Input: dimensioned drawing with shaded views. Units: mm. Origin: part minimum x, y, z. Give positions to 0.01 mm unless a question says otherwise; leave off trailing zeros. Order: outer loops, then holes, each group sorted by start corner. A loop starts at its lowest first (then second) coordinate and runs counter-clockwise, first axis right, second up. Notation, with made-up numbers: M 52.25,80.5 L 69.25,80.5 A19 cw 69.25,95.5 Z; hole C 23,46 d4. An arc over 180 degrees is marked long. Answer in a Markdown table with one row per item. Add a question column.
(1) Section query A-A, the plane x = 22. Return loops of the section in (y, z).
(2) Material intervals for line 1 along Z through (x, y) = (22, 13.1); line 2 along Y through (x, z) = (6.75, 2); line 3 along X through (y, z) = (11.5, 6.25), sorted ascending.
(3) Pin query (flat end, axial travel): P1, Ø1.5, axis at y = 13, z = 4, coming from the -X side; P2, Ø2.5, axis at x = 19.5, z = 4, coming from the -Y side; P3, Ø2, axis at y = 4, z = 9, coming from the -X side; P4, Ø3, axis at y = 2.5, z = 7, coming from the -X side. Return the tip coordinate at first contact, or that it passes through.
(4) Section query D-D, the plane y = 11.75. Return loops of the section in (x, z), plus the area to 3 significant figures.
(5) Section query B-B, the plane z = 5. Return loops of the section in (x, y), plus the area to 3 significant figures.
(6) Section query C-C, the plane z = 3. Return loops of the section in (x, y).
(7) Mould query, pull axis X, two halves, no side actions, for the marked faces 1, 2, 3 and 4. Classes: pulls with the +X half, pulls with the -X half, needs draft (parallel to the pull), parting line crosses it, or undercut.
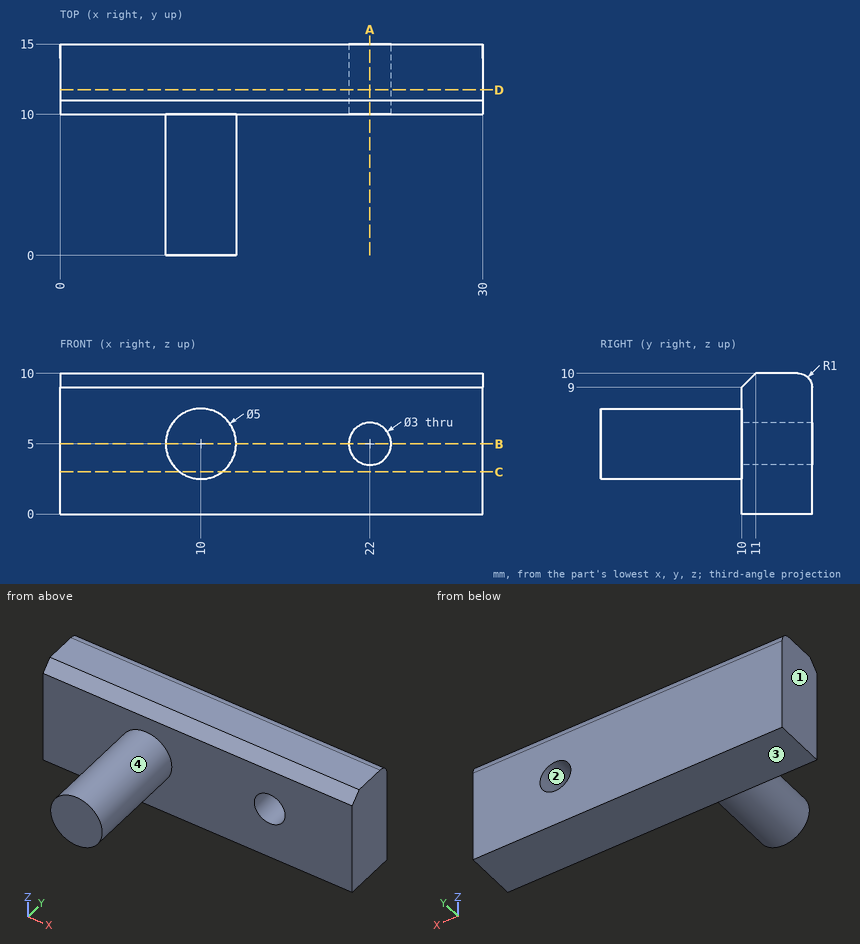
Values follow:
| question | item | result |
|---|---|---|
| 1 | outline | M 10,0 L 15,0 L 15,3.5 L 10,3.5 Z; M 10,6.5 L 15,6.5 L 15,9 A1 ccw 14,10 L 11,10 L 10,9 Z |
| 2 | line 1 | z = 0 to 3.5, 6.5 to 10 |
| 2 | line 2 | y = 10 to 15 |
| 2 | line 3 | x = 0 to 21.17, 22.83 to 30 |
| 3 | P1 | stops at x = 0 |
| 3 | P2 | stops at y = 10 |
| 3 | P3 | passes through |
| 3 | P4 | stops at x = 7.55 |
| 4 | outline | M 0,0 L 30,0 L 30,10 L 0,10 Z; hole C 22,5 d3 |
| 4 | area | 293 mm² |
| 5 | outline | M 0,10 L 7.5,10 L 7.5,0 L 12.5,0 L 12.5,10 L 20.5,10 L 20.5,15 L 0,15 Z; M 23.5,10 L 30,10 L 30,15 L 23.5,15 Z |
| 5 | area | 185 mm² |
| 6 | outline | M 0,10 L 8.5,10 L 8.5,0 L 11.5,0 L 11.5,10 L 30,10 L 30,15 L 0,15 Z |
| 7 | face 1 | pulls with the -X half |
| 7 | face 2 | undercut |
| 7 | face 3 | needs draft |
| 7 | face 4 | parting line crosses it |
